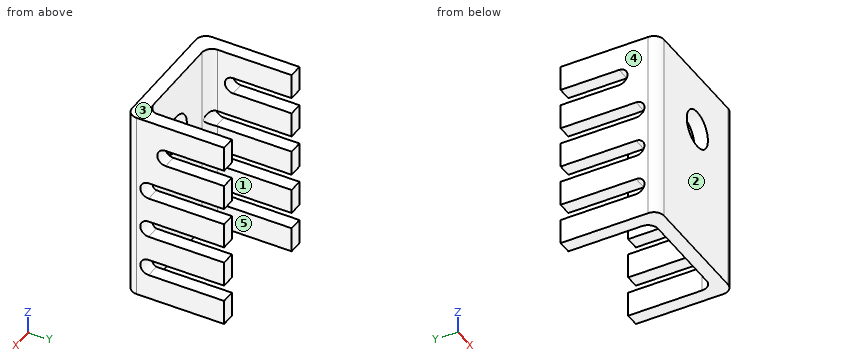
```python
from build123d import *

# Parameters (mm, degrees)
BOSS_EXTRUDE3_DEPTH = 19.1
CUT_EXTRUDE2_REACH  = 23.854
SKETCH3_R           = 1.85
CUT_EXTRUDE3_DEPTH  = 26.150723648


with BuildPart() as part:
    # Sketch1 → Boss-Extrude3 (new body)
    with BuildSketch(Plane.XY):
        with BuildLine():
            Line((-5.6, 0), (5.6, 0))
            ThreePointArc((5.6, 0), (6.307106781, 0.292893219), (6.6, 1))
            Line((6.6, 1), (6.6, 9.67))
            Line((6.6, 9.67), (5.25, 9.67))
            Line((5.25, 9.67), (5.25, 2.35))
            ThreePointArc((5.25, 2.35), (4.957106781, 1.642893219), (4.25, 1.35))
            Line((4.25, 1.35), (-4.25, 1.35))
            ThreePointArc((-4.25, 1.35), (-4.957106781, 1.642893219), (-5.25, 2.35))
            Line((-5.25, 2.35), (-5.25, 9.67))
            Line((-5.25, 9.67), (-6.6, 9.67))
            Line((-6.6, 9.67), (-6.6, 1))
            ThreePointArc((-6.6, 1), (-6.307106781, 0.292893219), (-5.6, 0))
        make_face()
    extrude(amount=-BOSS_EXTRUDE3_DEPTH)

    # Sketch3 → Cut-Extrude2 (cut, up to next)
    with BuildSketch(Plane(origin=(0, 1.35, 0), x_dir=(1, 0, 0), z_dir=(0, 1, 0)), mode=Mode.PRIVATE) as cut_extrude2_sk1:
        with Locations(Location((0.241401012, 5.85, 0), (0, 0, 270))):
            Circle(SKETCH3_R)
    cut_extrude2_tool1 = extrude(cut_extrude2_sk1.sketch, amount=-CUT_EXTRUDE2_REACH, mode=Mode.PRIVATE) & part.part
    add(cut_extrude2_tool1.solids().sort_by_distance((0.241401, 1.35, -5.85))[0], mode=Mode.SUBTRACT)

    # Sketch4 → Cut-Extrude3 (cut, through all)
    with BuildSketch(Plane(origin=(6.6, 0, 0), x_dir=(0, 0, -1), z_dir=(1, 0, 0))):
        with BuildLine():
            Line((2.5, 9.67), (2.5, 3.88))
            ThreePointArc((2.5, 3.88), (3.325, 3.055), (4.15, 3.88))
            Line((4.15, 3.88), (4.15, 9.67))
            Line((4.15, 9.67), (2.5, 9.67))
        make_face()
        with BuildLine():
            Line((6.65, 9.67), (6.65, 2.2))
            ThreePointArc((6.65, 2.2), (7.475, 1.375), (8.3, 2.2))
            Line((8.3, 2.2), (8.3, 9.67))
            Line((8.3, 9.67), (6.65, 9.67))
        make_face()
        with BuildLine():
            Line((10.8, 9.67), (10.8, 2.2))
            ThreePointArc((10.8, 2.2), (11.625, 1.375), (12.45, 2.2))
            Line((12.45, 2.2), (12.45, 9.67))
            Line((12.45, 9.67), (10.8, 9.67))
        make_face()
        with BuildLine():
            Line((14.95, 9.67), (14.95, 2.2))
            ThreePointArc((14.95, 2.2), (15.775, 1.375), (16.6, 2.2))
            Line((16.6, 2.2), (16.6, 9.67))
            Line((16.6, 9.67), (14.95, 9.67))
        make_face()
    extrude(amount=-CUT_EXTRUDE3_DEPTH, mode=Mode.SUBTRACT)


solid = part.part
```
The listing builds one solid part. Answer for the finished solid, in the listing's coordinates (mm). Face numbers are marked on the shaded views. A direction names the side the tool comes from. Round coordinates to 2 decimals unless told otherwise and drop trailing zeros. Loops run counter-clockwise (first coordinate to the right, second up) from the corner with the lowest first, then second, coordinate; pieces in that order, holes last. Notation, with made-up numbers: (70, 47.25) - (98, 47.25) arc R21 ccw to (98, 83.25) - close; hole circle Ø8 at (-16.75, -14.5). An arc over 180 degrees is marked (long way). Use one line per item in the form item = value. Start each with the question number.
1. For a pull along X with two mould halves and no side action, classify the marked faces 3, 4 and 5 as pulls with the +X half, pulls with the -X half, needs draft (parallel to the pull), parting line crosses it, or undercut.
2. Given pin 1 Ø1 at (x, z) = (-3.5, -12) entering from +Y, flat-ended and moving along its own axis, determine where the tip first touches the part or whether it passes through.
3. The part is cut by section A-A on z = -5.85. Determine the outline of the cut face in (x, y), then the cut area to 3 significant figures.
4. A tool of negligible diameter and unlimited length cuts with its end or side. For the marked faces 1 and 2, from which of +Z, -Z, +X, -X, +Y, -Y can it reach the whole face along a straight path? Write none if from no direction.
5. The part is cut by section B-B on x = -1.25. Determine the outline of the cut face in (y, z), then the cut area to 3 significant figures.
6. The part is cut by section C-C on y = 6.25. Give the number of separate pieces and of enclosed holes in the cut face, then the cut area to 4 significant figures.
7. Consider line 1 (Z direction, x = 5.75, y = 2.5); line 2 (X direction, y = 6, z = -6); line 3 (Z direction, x = 6, y = 7). Determine where each line is inside the solid, lowest interval first. Write a range as [from, to].
8. The part is cut by section D-D on z = -14. Determine the outline of the cut face in (x, y), then the cut area to 3 significant figures.
Geometry check:
q1.face_3 = needs draft
q1.face_4 = pulls with the -X half
q1.face_5 = undercut
q2.pin_1 = 1.35
q3.outline = (-6.6, 1) arc R1 ccw to (-5.6, 0) - (-1.61, 0) - (-1.61, 1.35) - (-4.25, 1.35) arc R1 cw to (-5.25, 2.35) - (-5.25, 9.67) - (-6.6, 9.67) - close; (2.09, 0) - (5.6, 0) arc R1 ccw to (6.6, 1) - (6.6, 9.67) - (5.25, 9.67) - (5.25, 2.35) arc R1 cw to (4.25, 1.35) - (2.09, 1.35) - close
q3.area = 35.3 mm^2
q4.face_1 = +Z, -Z, +Y
q4.face_2 = +Z, -Z, +X, -X, -Y
q5.outline = (0, -19.1) - (1.35, -19.1) - (1.35, -6.94) - (0, -6.94) - close; (0, -4.76) - (1.35, -4.76) - (1.35, 0) - (0, 0) - close
q5.area = 22.8 mm^2
q6.separate_pieces = 10
q6.enclosed_holes = 0
q6.area = 33.75 mm^2
q7.line_1 = [-19.1, -16.6], [-14.95, -12.45], [-10.8, -8.3], [-6.65, 0]
q7.line_2 = [-6.6, -5.25], [5.25, 6.6]
q7.line_3 = [-19.1, -16.6], [-14.95, -12.45], [-10.8, -8.3], [-6.65, -4.15], [-2.5, 0]
q8.outline = (-6.6, 1) arc R1 ccw to (-5.6, 0) - (5.6, 0) arc R1 ccw to (6.6, 1) - (6.6, 9.67) - (5.25, 9.67) - (5.25, 2.35) arc R1 cw to (4.25, 1.35) - (-4.25, 1.35) arc R1 cw to (-5.25, 2.35) - (-5.25, 9.67) - (-6.6, 9.67) - close
q8.area = 40.3 mm^2
